Build history of the part. All positions in model axes, mm. Round coordinates to 2 decimals unless told otherwise and drop trailing zeros. Write each loop counter-clockwise with the first axis right and the second up, starting at its lowest first coordinate (ties: lowest second). Pieces come first, ordered by that corner, then holes. Notation, with made-up numbers: (46, 22) - (99, 22) arc R23 ccw to (99, 40) - close; hole circle Ø2 at (74.5, 30). An arc over 180 degrees is marked (long way). One line per question, with ' | ' between items.
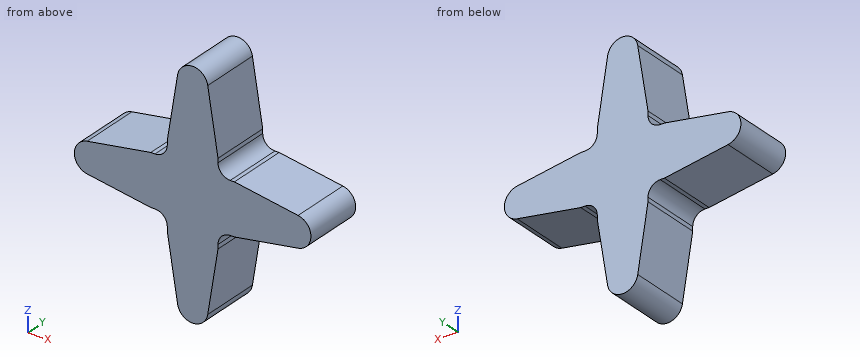
from build123d import *

# Parameters (mm, degrees)
PAD_DEPTH = 10


with BuildPart() as part:
    # Sketch → Pad (new body)
    with BuildSketch(Plane.XZ):
        with BuildLine():
            Line((-6.836766, 4.15), (-6.15, 4.15))
            ThreePointArc((-6.15, 4.15), (-4.735786, 4.735786), (-4.15, 6.15))
            Line((-4.15, 6.15), (-4.15, 6.836766))
            Line((-4.15, 6.836766), (-2.468004, 17.248694))
            ThreePointArc((2.468004, 17.248694), (0, 19.35), (-2.468004, 17.248694))
            Line((2.468004, 17.248694), (4.15, 6.836766))
            Line((4.15, 6.836766), (4.15, 6.15))
            ThreePointArc((4.15, 6.15), (4.735786, 4.735786), (6.15, 4.15))
            Line((6.15, 4.15), (6.836766, 4.15))
            Line((6.836766, 4.15), (17.248715, 2.468004))
            ThreePointArc((17.248715, -2.468004), (19.350021, 0), (17.248715, 2.468004))
            Line((17.248715, -2.468004), (6.836766, -4.15))
            Line((6.836766, -4.15), (6.15, -4.15))
            ThreePointArc((6.15, -4.15), (4.735786, -4.735786), (4.15, -6.15))
            Line((4.15, -6.15), (4.15, -6.836766))
            Line((4.15, -6.836766), (2.468004, -17.248694))
            ThreePointArc((-2.468004, -17.248694), (0, -19.35), (2.468004, -17.248694))
            Line((-2.468004, -17.248694), (-4.15, -6.836766))
            Line((-4.15, -6.836766), (-4.15, -6.15))
            ThreePointArc((-4.15, -6.15), (-4.735786, -4.735786), (-6.15, -4.15))
            Line((-6.15, -4.15), (-6.836766, -4.15))
            Line((-6.836766, -4.15), (-17.248715, -2.468004))
            ThreePointArc((-17.248715, 2.468004), (-19.350021, 0), (-17.248715, -2.468004))
            Line((-17.248715, 2.468004), (-6.836766, 4.15))
        make_face()
    extrude(amount=PAD_DEPTH)


solid = part.part
Q1. Saw through at C-C, the plane x = -15. List the corners of the cut face in (y, z).
Found:
outline: (-10, -2.83) - (0, -2.83) - (0, 2.83) - (-10, 2.83) - close
Q2. Drill centre lines: L1, parallel to X at y = -3.5, z = 11.5; L2, parallel to Z at x = -4.5, y = -3.25; L3, parallel to Z at x = 6.5, y = -2.5. Where is each one in solid material? Low to high. Write a range as from..to.
Found:
L1: -3.4..3.4 | L2: -5.02..5.02 | L3: -4.15..4.15
Q3. Saw through at B-B, the plane z = -16.5. List the corners of the cut face in (x, y), then the cut area to 3 significant figures.
Found:
outline: (-2.59, -10) - (2.59, -10) - (2.59, 0) - (-2.59, 0) - close | area: 51.8 mm^2
Q4. Saw through at A-A, the plane y = -5.75. List the corners of the cut face in (x, z), then the cut area to 3 significant figures.
Found:
outline: (-17.25, -2.47) - (-6.84, -4.15) - (-6.15, -4.15) arc R2 cw to (-4.15, -6.15) - (-4.15, -6.84) - (-2.47, -17.25) arc R2.5 ccw to (2.47, -17.25) - (4.15, -6.84) - (4.15, -6.15) arc R2 cw to (6.15, -4.15) - (6.84, -4.15) - (17.25, -2.47) arc R2.5 ccw to (17.25, 2.47) - (6.84, 4.15) - (6.15, 4.15) arc R2 cw to (4.15, 6.15) - (4.15, 6.84) - (2.47, 17.25) arc R2.5 ccw to (-2.47, 17.25) - (-4.15, 6.84) - (-4.15, 6.15) arc R2 cw to (-6.15, 4.15) - (-6.84, 4.15) - (-17.25, 2.47) arc R2.5 ccw to start | area: 468 mm^2
Q5. Drop flat-ended pins along their axis: pin 1 (12 mm diameter, centred on x = -10, z = 10.5, fed in from -Y); pin 2 (1.5 mm diameter, centred on y = -7, z = -5.5, fed in from +X); pin 3 (0.5 mm diameter, centred on y = -6, z = -6.5, fed in from -X); pin 4 (1 mm diameter, centred on x = -12, z = 2, fed in from +Y). Give the stop position or say it passes through.
Found:
pin 1: through | pin 2: x = 4.72 | pin 3: x = -4.15 | pin 4: y = 0
